Can you work these out from the model? Positions are in its coordinate system, mm. A direction names the side the tool comes from. Give positions to 0.01 mm unless a question says otherwise; leave off trailing zeros. Write each loop counter-clockwise with the first axis right and the second up, starting at its lowest first coordinate (ties: lowest second). Pieces come first, ordered by that corner, then holes.
1. Suppose I cut it at D-D (x = -44.45). Please give me the cut outline in (y, z) (3 decimals), and give its area (3 significant figures).
2. Suppose I cut it at A-A (z = 0). Please give me the cut outline in (x, y) (3 decimals).
3. On a 3-axis mill with a long thin cutter (end or side, diameter ignored), from which of +Z, -Z, +X, -X, +Y, -Y can I reach the whole of each face in a straight line? I mean faces 1 (the cylindrical face through (117.473, 10.957, 0.694)), 2 (the cylindrical face through (0.911, 10.957, 46.035)). Say none if no direction works.
4. I'm going to push flat-ended pins straight in: pin 1 (5 mm diameter, centred on y = 3, z = 21.5, fed in from +X); pin 2 (12 mm diameter, centred on x = 37, y = 9, fed in from +Z); pin 3 (12 mm diameter, centred on y = 5.5, z = 58.5, fed in from -X); pin 4 (11.5 mm diameter, centred on x = -103.19, z = 0, fed in from -Y). Where does each tip first touch, or does it pass through?
5. Suppose I cut it at B-B (x = -0.5). Please give me the cut outline in (y, z) (3 decimals), and give its area (3 significant figures).
6. If I drill on probe 1 along X at (y, z) = (14.5, 0) (3 decimals); probe 2 along Z at (x, y) = (44.45, 10); probe 3 along X at (y, z) = (18, -72.5), over which ranges is the centre line in solid material (lowest first)?
7. Suppose I cut it at C-C (y = 19.25). Give the number of separate pieces and of enclosed holes in the cut face, and give its area (3 significant figures).
8. Thinking about a two-plate mould opening in X: for faces 3 (the cylindrical face through (-73.024, 10.957, 0.431)), 4 (the cylindrical face through (43.52, 10.96, 62.27)), 5 (the cylindrical face through (-117.473, 10.957, -0.694)), 6 (the flat face through (-2, 22.225, -62)), which applies, pulls with the +X half, pulls with the -X half, needs draft (parallel to the pull), parting line crosses it, or undercut?
```python
from build123d import *

# Parameters (mm, degrees)
SKETCH1_R           = 7.14375
BOSS_EXTRUDE1_DEPTH = 22.225


with BuildPart() as part:
    # Sketch1 → Boss-Extrude1 (new body)
    with BuildSketch(Plane(origin=(0, 0, 0), x_dir=(1, 0, 0), z_dir=(0, 1, 0))):
        with BuildLine():
            ThreePointArc((80.690921224, 74.058849944), (0, 90.4875), (-80.690921224, 74.058849944))
            ThreePointArc((-80.690921224, 74.058849944), (-96.385165084, 63.584590133), (-107.174095369, 48.104977984))
            ThreePointArc((-107.174095369, 48.104977984), (-117.475, 0), (-107.174095369, -48.104977984))
            ThreePointArc((-107.174095369, -48.104977984), (-96.385165084, -63.584590133), (-80.690921224, -74.058849944))
            ThreePointArc((-80.690921224, -74.058849944), (0, -90.4875), (80.690921224, -74.058849944))
            ThreePointArc((80.690921224, -74.058849944), (96.385165084, -63.584590133), (107.174095369, -48.104977984))
            ThreePointArc((107.174095369, -48.104977984), (117.475, 0), (107.174095369, 48.104977984))
            ThreePointArc((107.174095369, 48.104977984), (96.385165084, 63.584590133), (80.690921224, 74.058849944))
        make_face()
        with Locations((-103.1875, 0)):
            Circle(SKETCH1_R, mode=Mode.SUBTRACT)
        with Locations((-44.45, 69.354092252)):
            Circle(SKETCH1_R, mode=Mode.SUBTRACT)
        with Locations((103.1875, 0)):
            Circle(SKETCH1_R, mode=Mode.SUBTRACT)
        with Locations((44.45, 69.354092252)):
            Circle(SKETCH1_R, mode=Mode.SUBTRACT)
        with Locations((-44.45, -69.354092252)):
            Circle(SKETCH1_R, mode=Mode.SUBTRACT)
        with Locations((44.45, -69.354092252)):
            Circle(SKETCH1_R, mode=Mode.SUBTRACT)
        with BuildLine():
            ThreePointArc((-66.621734959, -29.903094423), (-73.025, 0), (-66.621734959, 29.903094423))
            ThreePointArc((-66.621734959, 29.903094423), (-65.273118673, 31.838045941), (-63.311338191, 33.147328418))
            ThreePointArc((-63.311338191, 33.147328418), (0, 46.0375), (63.311338191, 33.147328418))
            ThreePointArc((63.311338191, 33.147328418), (65.273118673, 31.838045941), (66.621734959, 29.903094423))
            ThreePointArc((66.621734959, 29.903094423), (73.025, 0), (66.621734959, -29.903094423))
            ThreePointArc((66.621734959, -29.903094423), (65.273118673, -31.838045941), (63.311338191, -33.147328418))
            ThreePointArc((63.311338191, -33.147328418), (0, -46.0375), (-63.311338191, -33.147328418))
            ThreePointArc((-63.311338191, -33.147328418), (-65.273118673, -31.838045941), (-66.621734959, -29.903094423))
        make_face(mode=Mode.SUBTRACT)
    extrude(amount=BOSS_EXTRUDE1_DEPTH)


solid = part.part
```
Checks:
1. outline: (0, -85.644) - (22.225, -85.644) - (22.225, -76.498) - (0, -76.498) - close; (0, -62.21) - (22.225, -62.21) - (22.225, -39.817) - (0, -39.817) - close; (0, 39.817) - (22.225, 39.817) - (22.225, 62.21) - (0, 62.21) - close; (0, 76.498) - (22.225, 76.498) - (22.225, 85.644) - (0, 85.644) - close
1. area: 1,400 mm2
2. outline: (-117.475, 0) - (-110.331, 0) - (-110.331, 22.225) - (-117.475, 22.225) - close; (-96.044, 0) - (-73.025, 0) - (-73.025, 22.225) - (-96.044, 22.225) - close; (73.025, 0) - (96.044, 0) - (96.044, 22.225) - (73.025, 22.225) - close; (110.331, 0) - (117.475, 0) - (117.475, 22.225) - (110.331, 22.225) - close
3. face 1: +X, +Y, -Y
3. face 2: +Y, -Y
4. pin 1: stops at x = 115.93
4. pin 2: stops at z = 88.15
4. pin 3: stops at x = -104.94
4. pin 4: passes through
5. outline: (0, -90.487) - (22.225, -90.487) - (22.225, -46.037) - (0, -46.037) - close; (0, 46.037) - (22.225, 46.037) - (22.225, 90.487) - (0, 90.487) - close
5. area: 1,980 mm2
6. probe 1: x = -117.475 to -110.331, -96.044 to -73.025, 73.025 to 96.044, 110.331 to 117.475
6. probe 2: z = -85.64 to -76.5, -62.21 to -39.82, 39.82 to 62.21, 76.5 to 85.64
6. probe 3: x = -84.02 to -50.86, -38.04 to 38.04, 50.86 to 84.02
7. separate pieces: 1
7. enclosed holes: 7
7. area: 23,100 mm2
8. face 3: undercut
8. face 4: undercut
8. face 5: pulls with the -X half
8. face 6: needs draft
